Can you work these out from the model? Positions are in its coordinate system, mm. A direction names the side the tool comes from. Give positions to 0.01 mm unless a question says otherwise; leave off trailing zeros. Order: outer loops, then holes, each group sorted by start corner. A loop starts at its lowest first (then second) coordinate and runs counter-clockwise, first axis right, second up.
Item 1: Which directions (+Z, -Z, +X, -X, +Y, -Y) give clear straight access to the entire face, cutting with the end or side of a thin tool? Please do faces 1 (the flat face through (0, -3, -2.388)), 2 (the flat face through (2.35, 0, 0)).
Item 2: I want a section at A-A, the plane y = -3. Write out the boundary of the cut face in (x, z), then the cut area to 3 significant figures.
Item 3: I want a section at B-B, the plane x = 1.05. Write out the boundary of the cut face in (y, z), then the cut area to 3 significant figures.
Item 4: I want a section at C-C, the plane z = 0.5. Write out the boundary of the cut face in (x, y), then the cut area to 3 significant figures.
Item 5: If we mould it in two halves opening along Z, with no side actions, what happens to faces 3 (the flat face through (0, -3, 1.575)), 4 (the flat face through (0, 0, -29.362)), 5 (the flat face through (0, -4.318, 16))? For each: +Z half, -Z half, draft (parallel to the pull), parting line (faces both ways), or undercut.
Item 6: If I drill on line 1 along Z through (x, y) = (1.4, -2.5); line 2 along Y through (x, z) = (0.6, -1.5), over which ranges is the centre line in solid material (lowest first)?
```python
from build123d import *

# Parameters (mm, degrees)
SKETCH1_W               = 58.7248
SKETCH1_H               = 8.636
BOSS_EXTRUDE1_DEPTH     = 2.3495
CUT_EXTRUDE1_DEPTH      = 31.047899407
CUT_EXTRUDE1_DEPTH_BACK = 31.047899407
SKETCH2_W               = 3.9624
SKETCH2_H               = 3.175


with BuildPart() as part:
    # Sketch1 → Boss-Extrude1 (new, symmetric)
    with BuildSketch(Plane(origin=(0, 0, 0), x_dir=(0, 0, -1), z_dir=(1, 0, 0))):
        Rectangle(SKETCH1_W, SKETCH1_H)
    extrude(amount=BOSS_EXTRUDE1_DEPTH, both=True)

    # Sketch2 → Cut-Extrude1 (cut, two sides: drawn at the far end of the back side and taken through both)
    with BuildSketch(Plane(origin=(2.3495, 0, 0), x_dir=(0, 0, -1), z_dir=(1, 0, 0)).offset(-CUT_EXTRUDE1_DEPTH_BACK)):
        with Locations((0.4064, -2.7305)):
            Rectangle(SKETCH2_W, SKETCH2_H)
    extrude(amount=CUT_EXTRUDE1_DEPTH + CUT_EXTRUDE1_DEPTH_BACK, mode=Mode.SUBTRACT)


solid = part.part
```
Results list:
1. face 1: +X, -X, -Y
1. face 2: +Z, -Z, +X, +Y, -Y
2. outline: (-2.35, -29.36) - (2.35, -29.36) - (2.35, -2.39) - (-2.35, -2.39) - close; (-2.35, 1.57) - (2.35, 1.57) - (2.35, 29.36) - (-2.35, 29.36) - close
2. area: 257 mm2
3. outline: (-4.32, -29.36) - (4.32, -29.36) - (4.32, 29.36) - (-4.32, 29.36) - (-4.32, 1.57) - (-1.14, 1.57) - (-1.14, -2.39) - (-4.32, -2.39) - close
3. area: 495 mm2
4. outline: (-2.35, -1.14) - (2.35, -1.14) - (2.35, 4.32) - (-2.35, 4.32) - close
4. area: 25.7 mm2
5. face 3: undercut
5. face 4: -Z half
5. face 5: draft
6. line 1: z = -29.36 to -2.39, 1.57 to 29.36
6. line 2: y = -1.14 to 4.32
